Here's the drawing with two shaded views (mm, measured from the low corner). I have some questions. Give positions to 0.01 mm unless a question says otherwise; leave off trailing zeros. Write each loop counter-clockwise with the first axis right and the second up, starting at its lowest first coordinate (ties: lowest second). Pieces come first, ordered by that corner, then holes. Notation, with made-up numbers: (46.25, 22.5) - (65.25, 22.5) arc R25 cw to (65.25, 34.5) - close; hole circle Ø1 at (24.5, 59). An arc over 180 degrees is marked (long way). Answer as a JSON object with one key per item and string values. Group by question number.
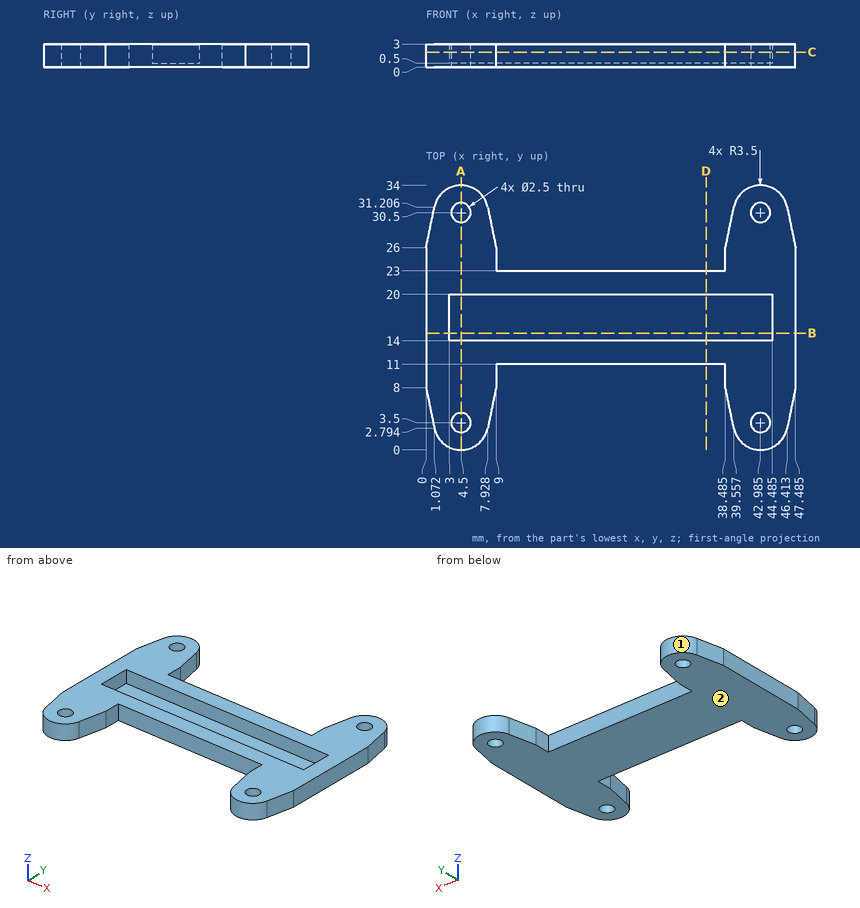
(1) If we mould it in two halves opening along X, with no side actions, what happens to the marked faces 1 and 2? For each: +X half, -X half, draft (parallel to the pull), parting line (faces both ways), or undercut.
(2) I want a section at C-C, the plane z = 1.95. State how many separate pieces and enclosed holes the cut face has, and give its area (3 significant figures).
(3) I want a section at D-D, the plane x = 36. Please give me the cut outline in (y, z).
(4) I need wall thicknesses on L1, parallel to Y at x = 24, z = 0.85; L2, parallel to X at y = 4, z = 0.8 (1 decimal); L3, parallel to X at y = 18, z = 0.65 (1 decimal). Which ranges of each line are inside material? Lowest first, please.
(5) Will these pins go through, and if not, where does the flat tip stop? P1, Ø1.2, axis at x = 30.5, z = 1.5, coming from the +Y side; P2, Ø2, axis at x = 42.99, y = 3.5, coming from the -Z side; P3, Ø1.5, axis at x = 18.5, z = 1.5, coming from the -Y side.
(6) I want a section at B-B, the plane y = 15. Please give me the cut outline in (x, z) (1 decimal).
(7) I want a section at A-A, the plane x = 4.5. Please give me the cut outline in (y, z), and give its area (3 significant figures).
Entries:
{
 "1": {"face 1": "undercut", "face 2": "draft"},
 "2": {"separate pieces": "1", "enclosed holes": "5", "area": "632 mm^2"},
 "3": {"outline": "(11, 0) - (23, 0) - (23, 3) - (20, 3) - (20, 0.5) - (14, 0.5) - (14, 3) - (11, 3) - close"},
 "4": {"L1": "11 to 14, 20 to 23", "L2": "0.8 to 3.4, 5.6 to 8.2, 39.3 to 41.8, 44.1 to 46.7", "L3": "0 to 3, 44.5 to 47.5"},
 "5": {"P1": "y = 23", "P2": "through", "P3": "y = 11"},
 "6": {"outline": "(0, 0) - (47.5, 0) - (47.5, 3) - (44.5, 3) - (44.5, 0.5) - (3, 0.5) - (3, 3) - (0, 3) - close"},
 "7": {"outline": "(0, 0) - (2.25, 0) - (2.25, 3) - (0, 3) - close; (4.75, 0) - (29.25, 0) - (29.25, 3) - (20, 3) - (20, 0.5) - (14, 0.5) - (14, 3) - (4.75, 3) - close; (31.75, 0) - (34, 0) - (34, 3) - (31.75, 3) - close", "area": "72.0 mm^2"}
}
